The listing builds one solid part. Answer for the finished solid, in the listing's coordinates (mm). A direction names the side the tool comes from. Round coordinates to 2 decimals unless told otherwise and drop trailing zeros. Loops run counter-clockwise (first coordinate to the right, second up) from the corner with the lowest first, then second, coordinate; pieces in that order, holes last. Notation, with made-up numbers: (48.25, -36.75) -> (100.25, -36.75) arc R11 ccw to (100.25, -28.75) -> close; hole circle Ø8 at (7.25, -26.75). An arc over 180 degrees is marked (long way). One line per question, with ' | ' between items.
from build123d import *

# Parameters (mm, degrees)
BOX006_W               = 6
BOX006_H               = 30
BOX006_DEPTH           = 10
FILLET007_R            = 2
BOX002_W               = 10
BOX002_H               = 100
BOX002_DEPTH           = 10
BOX002_PLACEMENT_ANGLE = -27
BOX001_W               = 10
BOX001_H               = 100
BOX001_DEPTH           = 10
BOX001_PLACEMENT_ANGLE = 27
BOX_W                  = 40
BOX_H                  = 52
BOX_DEPTH              = 10
FILLET_R               = 5
FILLET001_R            = 2
FILLET002_R            = 2
BOX005_W               = 10
BOX005_H               = 100
BOX005_DEPTH           = 10
BOX005_PLACEMENT_ANGLE = 27
BOX004_W               = 10
BOX004_H               = 100
BOX004_DEPTH           = 10
BOX004_PLACEMENT_ANGLE = -27
BOX003_W               = 44
BOX003_H               = 56
BOX003_DEPTH           = 7
FILLET003_R            = 7
FILLET004_R            = 3
FILLET005_R            = 3
FILLET006_R            = 1


with BuildPart() as fillet007:
    # Box006 → Box006 (new body)
    with BuildSketch(Plane(origin=(17, 30, 0), x_dir=(1, 0, 0), z_dir=(0, 0, 1))):
        with Locations((3, 15)):
            Rectangle(BOX006_W, BOX006_H)
    extrude(amount=BOX006_DEPTH)

    # Fillet007
    fillet007_edges = [fillet007.edges().sort_by_distance(p)[0] for p in [
        (17, 45, 0),
        (23, 45, 0),
    ]]
    fillet(fillet007_edges, radius=FILLET007_R)


with BuildPart() as fillet007_1:
    # Fillet007 placement: moved
    add(fillet007.part.moved(Location((0, 0, 4))))


with BuildPart() as cube002:
    # Box002 → Box002 (new body)
    with BuildSketch(Plane.XY):
        with Locations((5, 50)):
            Rectangle(BOX002_W, BOX002_H)
    extrude(amount=BOX002_DEPTH)


with BuildPart() as cube002_1:
    # Box002 placement: moved
    add(cube002.part.moved(Location((30, -9.5, 0))).rotate(Axis((30, -9.5, 0), (0, 0, 1)), BOX002_PLACEMENT_ANGLE))


with BuildPart() as cube001:
    # Box001 → Box001 (new body)
    with BuildSketch(Plane.XY):
        with Locations((5, 50)):
            Rectangle(BOX001_W, BOX001_H)
    extrude(amount=BOX001_DEPTH)


with BuildPart() as cube001_1:
    # Box001 placement: moved
    add(cube001.part.moved(Location((-1, -10, 0))).rotate(Axis((-1, -10, 0), (0, 0, 1)), BOX001_PLACEMENT_ANGLE))


with BuildPart() as gps_profile:
    # Box → Box (new body)
    with BuildSketch(Plane.XY):
        with Locations((20, 26)):
            Rectangle(BOX_W, BOX_H)
    extrude(amount=BOX_DEPTH)

    # Fillet
    fillet_edges = [gps_profile.edges().sort_by_distance(p)[0] for p in [
        (0, 52, 5),
        (40, 52, 5),
    ]]
    fillet(fillet_edges, radius=FILLET_R)

    # Cut: cut Cube001
    add(cube001_1.part, mode=Mode.SUBTRACT)

    # Cut001: cut Cube002
    add(cube002_1.part, mode=Mode.SUBTRACT)

    # Fillet001
    fillet001_edges = [gps_profile.edges().sort_by_distance(p)[0] for p in [
        (5.128008, 0, 5),
        (34.840492, 0, 5),
    ]]
    fillet(fillet001_edges, radius=FILLET001_R)

    # Fillet002
    fillet002_edges = [gps_profile.edges().sort_by_distance(p)[0] for p in [
        (40, 10.126105, 5),
        (0, 10.064282, 5),
    ]]
    fillet(fillet002_edges, radius=FILLET002_R)


with BuildPart() as gps_profile_1:
    # Fillet002 placement: moved
    add(gps_profile.part.moved(Location((0, 0, 1.5))))


with BuildPart() as cube005:
    # Box005 → Box005 (new body)
    with BuildSketch(Plane.XY):
        with Locations((5, 50)):
            Rectangle(BOX005_W, BOX005_H)
    extrude(amount=BOX005_DEPTH)


with BuildPart() as cube005_1:
    # Box005 placement: moved
    add(cube005.part.moved(Location((-3, -10, 0))).rotate(Axis((-3, -10, 0), (0, 0, 1)), BOX005_PLACEMENT_ANGLE))


with BuildPart() as cube004:
    # Box004 → Box004 (new body)
    with BuildSketch(Plane.XY):
        with Locations((5, 50)):
            Rectangle(BOX004_W, BOX004_H)
    extrude(amount=BOX004_DEPTH)


with BuildPart() as cube004_1:
    # Box004 placement: moved
    add(cube004.part.moved(Location((30, -13.5, 0))).rotate(Axis((30, -13.5, 0), (0, 0, 1)), BOX004_PLACEMENT_ANGLE))


with BuildPart() as gps_mount:
    # Box003 → Box003 (new body)
    with BuildSketch(Plane(origin=(-2, -2, 0), x_dir=(1, 0, 0), z_dir=(0, 0, 1))):
        with Locations((22, 28)):
            Rectangle(BOX003_W, BOX003_H)
    extrude(amount=BOX003_DEPTH)

    # Fillet003
    fillet003_edges = [gps_mount.edges().sort_by_distance(p)[0] for p in [
        (-2, 54, 3.5),
        (42, 54, 3.5),
    ]]
    fillet(fillet003_edges, radius=FILLET003_R)

    # Cut002: cut Cube004
    add(cube004_1.part, mode=Mode.SUBTRACT)

    # Cut003: cut Cube005
    add(cube005_1.part, mode=Mode.SUBTRACT)

    # Fillet004
    fillet004_edges = [gps_mount.edges().sort_by_distance(p)[0] for p in [
        (4.147059, -2, 3.5),
        (35.859543, -2, 3.5),
    ]]
    fillet(fillet004_edges, radius=FILLET004_R)

    # Fillet005
    fillet005_edges = [gps_mount.edges().sort_by_distance(p)[0] for p in [
        (42, 10.051326, 3.5),
        (-2, 10.064282, 3.5),
    ]]
    fillet(fillet005_edges, radius=FILLET005_R)

    # Cut004: cut GPS Profile
    add(gps_profile_1.part, mode=Mode.SUBTRACT)

    # Fillet006
    fillet006_edges = [gps_mount.edges().sort_by_distance(p)[0] for p in [
        (39.18359, 4.52381, 7),
        (41.91711, 10.071226, 7),
        (35.588636, -1.55792, 7),
        (42, 28.885781, 7),
        (20.003301, -2, 7),
        (39.949747, 51.949747, 7),
        (4.417965, -1.55792, 7),
        (20, 54, 7),
        (0.819711, 4.530288, 7),
        (0.050253, 51.949747, 7),
        (-1.91711, 10.084182, 7),
        (-2, 28.892259, 7),
    ]]
    fillet(fillet006_edges, radius=FILLET006_R)

    # Cut005: cut Fillet007
    add(fillet007_1.part, mode=Mode.SUBTRACT)


solid = gps_mount.part
Q1. Find the intervals of material crossed by line 1 (Y direction, x = 21, z = 3.25); line 2 (X direction, y = 14, z = 5.25); line 3 (Z direction, x = 7.5, y = 13), in increasing order. Write a range as from..to.
Numbers:
line 1: -2..0, 52..54 | line 2: -2..0, 40..42 | line 3: 0..1.5
Q2. For a pull along X with two mould halves and no side action, classify faces 1 (the face through (20, 26, 0)), 2 (the face through (20, 0, 4)), 3 (the face through (41.915, 10.062, 2.958)) as pulls with the +X half, pulls with the -X half, needs draft (parallel to the pull), parting line crosses it, or undercut.
Numbers:
face 1: needs draft | face 2: undercut | face 3: pulls with the +X half
Q3. Given pin 1 Ø1.1 at (y, z) = (53, 6.5) entering from -X; pin 2 Ø1 at (x, y) = (19.5, 53) entering from +Z; pin 3 Ø1.5 at (x, y) = (15, 24.5) entering from +Z, each flat-ended and moving along its own axis, determine where each tip first touches the part or whether it passes through.
Numbers:
pin 1: x = 0.73 | pin 2: z = 4 | pin 3: z = 1.5
Q4. A cutting plane is placed at D-D on x = 22. Give the vertices of the cut face in (y, z).
Numbers:
outline: (-2, 0) -> (54, 0) -> (54, 4.27) -> (52, 4.27) -> (52, 1.5) -> (0, 1.5) -> (0, 7) -> (-1, 7) arc R1 ccw to (-2, 6) -> close
Q5. For faces 4 (the face through (5.3, 0.3, 4.3)), 5 (the face through (40, 51.9, 3)), 6 (the face through (17.57, 53.01, 4.6)), determine the directions among +Z, -Z, +X, -X, +Y, -Y from which every point of the face is accessible in a straight line to the end or side of a thin tool.
Numbers:
face 4: +Z | face 5: +Z, -Z, +X, +Y | face 6: +Z, +Y
Q6. A cutting plane is placed at B-B on x = 30.5. Give the vertices of the cut face in (y, z).
Numbers:
outline: (-2, 0) -> (54, 0) -> (54, 6) arc R1 ccw to (53, 7) -> (52, 7) -> (52, 1.5) -> (0, 1.5) -> (0, 7) -> (-1, 7) arc R1 ccw to (-2, 6) -> close
Q7. A cutting plane is placed at A-A on z = 2.5. Give the vertices of the cut face in (x, y), plus the area to 3 significant figures.
Numbers:
outline: (-2, 10.78) arc R3 ccw to (-1.67, 9.42) -> (3.31, -0.36) arc R3 ccw to (5.99, -2) -> (34.02, -2) arc R3 ccw to (36.69, -0.36) -> (41.67, 9.41) arc R3 ccw to (42, 10.77) -> (42, 47) arc R7 ccw to (35, 54) -> (5, 54) arc R7 ccw to (-2, 47) -> close; hole (0, 10.54) arc R2 ccw to (0.22, 9.64) -> (4.57, 1.09) arc R2 ccw to (6.35, 0) -> (33.61, 0) arc R2 ccw to (35.4, 1.09) -> (39.78, 9.7) arc R2 ccw to (40, 10.61) -> (40, 47) arc R5 ccw to (35, 52) -> (5, 52) arc R5 ccw to (0, 47) -> close | area: 351 mm^2
Q8. A cutting plane is placed at C-C on y = 41. Give the vertices of the cut face in (x, z).
Numbers:
outline: (-2, 0) -> (42, 0) -> (42, 6) arc R1 ccw to (41, 7) -> (40, 7) -> (40, 1.5) -> (0, 1.5) -> (0, 7) -> (-1, 7) arc R1 ccw to (-2, 6) -> close
